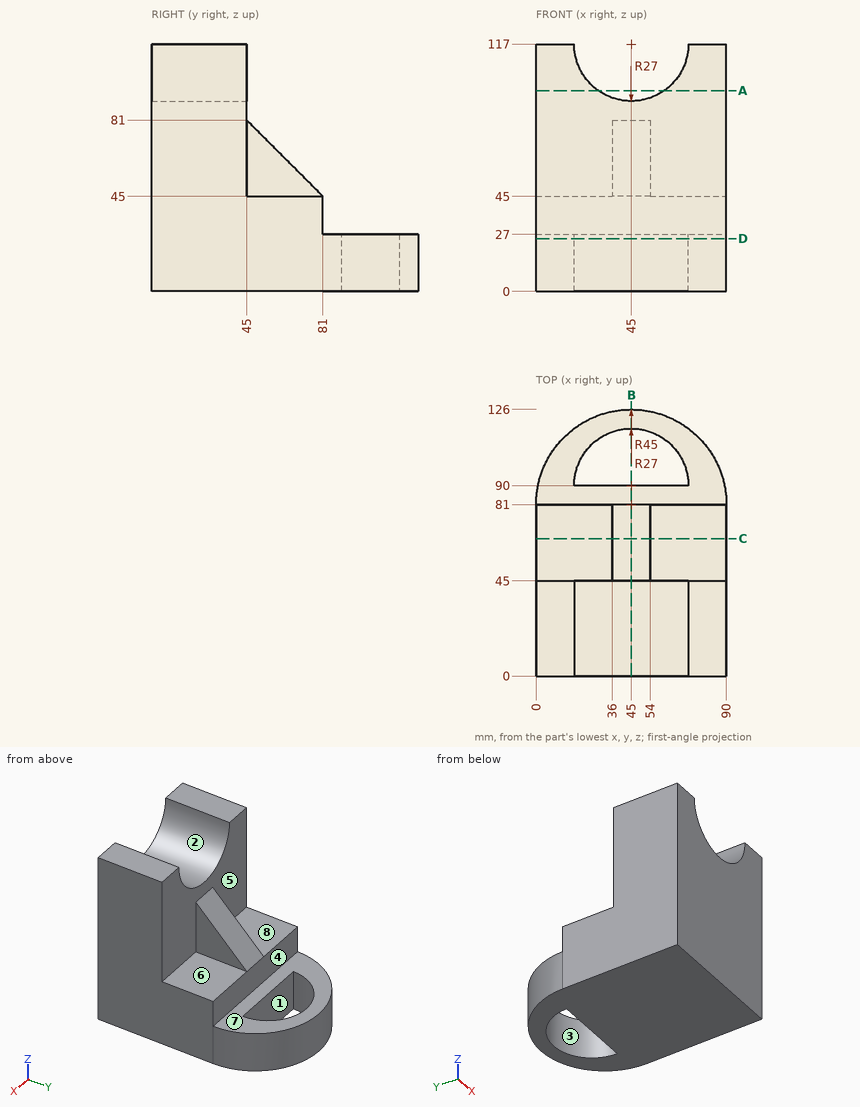
Part print with two shaded views. Sizes in mm from the minimum x, y, z corner. A direction names the side the tool comes from. Round coordinates to 2 decimals unless told otherwise and drop trailing zeros. Order: outer loops, then holes, each group sorted by start corner. A loop starts at its lowest first (then second) coordinate and runs counter-clockwise, first axis right, second up. Notation, with made-up numbers: M 58,-36 L 78,-36 A26 ccw 78,-12 Z; hole C 6,61 d1. An arc over 180 degrees is marked long. Answer in a Markdown table with one row per item. Add a question column.
Q1. Cut at D-D on z = 25. Give the cut face in (x, y).
Q2. 3-axis set-ups, long thin cutter, end or side, ignore diameter. For the marked faces 5, 6, 7 and 8: which of +Z, -Z, +X, -X, +Y, -Y reach the whole face in a straight line?
Q3. Pin check, flat tips, straight feed: pin 1 (11 mm diameter, centred on y = 68, z = 59, fed in from +X); pin 2 (21.5 mm diameter, centred on x = 41.5, z = 18, fed in from +Y); pin 3 (2 mm diameter, centred on x = 32.5, z = 52.5, fed in from +Y); pin 4 (12 mm diameter, centred on x = 48.5, y = 108, fed in from -Z). Stop position of each tip, or through.
Q4. Cut at C-C on y = 65. Give the cut face in (x, z), and give its area (3 significant figures).
Q5. Cut at A-A on z = 95. Give the cut face in (x, y).
Q6. Wall check: L1, parallel to X at y = 66, z = 58.5; L2, parallel to Y at x = 73, z = 68. Give the ranges that are in metal, low to high. Write a range as from..to.
Q7. Cut at B-B on x = 45. Give the cut face in (y, z), and give its area (3 significant figures).
Q8. Mould opens along Y. For the marked faces 1, 2, 3 and 4 say: +Y half, -Y half, draft (parallel to the pull), parting line (faces both ways), or undercut.
Established:
| question | item | result |
|---|---|---|
| 1 | outline | M 0,0 L 90,0 L 90,81 A45 ccw 0,81 Z; hole M 18,90 L 72,90 A27 ccw Z |
| 2 | face 5 | +Z, +Y |
| 2 | face 6 | +Z, +X, +Y |
| 2 | face 7 | +Z, +X, -X, +Y |
| 2 | face 8 | +Z, -X, +Y |
| 3 | pin 1 | stops at x = 54 |
| 3 | pin 2 | stops at y = 126 |
| 3 | pin 3 | stops at y = 45 |
| 3 | pin 4 | passes through |
| 4 | outline | M 0,0 L 90,0 L 90,45 L 54,45 L 54,61 L 36,61 L 36,45 L 0,45 Z |
| 4 | area | 4,340 mm2 |
| 5 | outline | M 0,0 L 29.35,0 L 29.35,45 L 0,45 Z; M 60.65,0 L 90,0 L 90,45 L 60.65,45 Z |
| 6 | L1 | x = 36..54 |
| 6 | L2 | y = 0..45 |
| 7 | outline | M 0,0 L 90,0 L 90,27 L 81,27 L 81,45 L 45,81 L 45,90 L 0,90 Z; M 117,0 L 126,0 L 126,27 L 117,27 Z |
| 7 | area | 6,800 mm2 |
| 8 | face 1 | undercut |
| 8 | face 2 | draft |
| 8 | face 3 | undercut |
| 8 | face 4 | +Y half |
